from build123d import *

# Parameters (mm, degrees)
SKETCH1_R           = 12.5
SKETCH1_R_2         = 5
BOSS_EXTRUDE1_DEPTH = 15
SKETCH2_R           = 15
SKETCH2_R_2         = 12.5
BOSS_EXTRUDE2_DEPTH = 10
RIB1_REACH          = 70.119
SKETCH3_WALL_W      = 146.04901068
SKETCH3_WALL_H      = 3
CIRPATTERN1_COUNT   = 3


with BuildPart() as part:
    # Sketch1 → Boss-Extrude1 (new body)
    with BuildSketch(Plane(origin=(0, 0, 0), x_dir=(0, 0, -1), z_dir=(1, 0, 0))):
        with BuildLine():
            Line((-41.109265282, -12.912706879), (-8.609265282, 42.087293121))
            ThreePointArc((-8.609265282, 42.087293121), (0, 47), (8.609265282, 42.087293121))
            Line((8.609265282, 42.087293121), (41.109265282, -12.912706879))
            ThreePointArc((41.109265282, -12.912706879), (41.185416835, -22.956161256), (32.5, -28))
            Line((32.5, -28), (-32.5, -28))
            ThreePointArc((-32.5, -28), (-41.185416835, -22.956161256), (-41.109265282, -12.912706879))
        make_face()
        Circle(SKETCH1_R, mode=Mode.SUBTRACT)
        with Locations((0, 37)):
            Circle(SKETCH1_R_2, mode=Mode.SUBTRACT)
        with Locations((32.5, -18)):
            Circle(SKETCH1_R_2, mode=Mode.SUBTRACT)
        with Locations((-32.5, -18)):
            Circle(SKETCH1_R_2, mode=Mode.SUBTRACT)
    extrude(amount=BOSS_EXTRUDE1_DEPTH)

    # Sketch2 → Boss-Extrude2 (add)
    with BuildSketch(Plane(origin=(15, 0, 0), x_dir=(0, 0, -1), z_dir=(1, 0, 0))):
        Circle(SKETCH2_R)
        Circle(SKETCH2_R_2, mode=Mode.SUBTRACT)
    extrude(amount=BOSS_EXTRUDE2_DEPTH)

    # Sketch3 wall → Rib1 (add, up to next)
    with BuildSketch(Plane(origin=(17.5, 18, 0), x_dir=(-0.640184399664, 0.768221279597, 0), z_dir=(-0.768221279597, -0.640184399664, 0)), mode=Mode.PRIVATE) as rib1_sk1:
        Rectangle(SKETCH3_WALL_W, SKETCH3_WALL_H)
    rib1_tool1 = extrude(rib1_sk1.sketch, amount=RIB1_REACH, mode=Mode.PRIVATE) - part.part
    rib1 = rib1_tool1.solids().sort_by_distance((17.5, 18, 0))[0]
    add(rib1)

    # CirPattern1: Rib1 ×3 about axis
    cirpattern1_axis = Axis((0, 0, 0), (1, 0, 0))
    for i in range(1, CIRPATTERN1_COUNT):
        add(rib1.rotate(cirpattern1_axis, i * 360 / CIRPATTERN1_COUNT))


solid = part.part
Verification items for the finished model (mm, model axes). A direction names the side the tool comes from. Give positions to 0.01 mm unless a question says otherwise; leave off trailing zeros. Order: outer loops, then holes, each group sorted by start corner. A loop starts at its lowest first (then second) coordinate and runs counter-clockwise, first axis right, second up. Notation, with made-up numbers: M 31.25,-18 L 49.25,-18 A26 ccw 49.25,8 Z; hole C -27,-12.75 d10. An arc over 180 degrees is marked long. Use one line per item in the form item = value. Start each with the question number.
Q1. Section check C-C (x = 12.25). Enter the section's corners in (y, z).
Q2. Section check B-B (z = 35.5). Enter the section's corners in (x, y), then the cut area to 3 significant figures.
Q3. Mould release check, pull along Y, two halves, no side actions. Record for faces 1 (the flat face through (7.395, 14.972, -24.632)), 2 (the flat face through (7, -28, 0)), 3 (the flat face through (16.758, -7.324, 15.685)): +Y half, -Y half, draft (parallel to the pull), parting line (faces both ways), or undercut.
Q4. Go/stop test with flat-tipped pins: pin 1 Ø13 at (y, z) = (37, 0) entering from +X; pin 2 Ø15 at (y, z) = (0, 0) entering from -X; pin 3 Ø5 at (x, y) = (14, -14.5) entering from +Z; pin 4 Ø4 at (x, y) = (16.5, 17.5) entering from -Z. Record where each tip stops, or that it passes through.
Q5. Access from +Z, -Z, +X, -X, +Y, -Y to the whole of each face (thin tool, end or side, straight path). Record for faces 4 (the flat face through (17, 17, 1.5)), 5 (the flat face through (16.758, -7.324, -15.685)), 6 (the flat face through (15, -15, 9)), 7 (the flat face through (17.567, -8.942, 15.53)), 8 (the flat face through (16.758, -9.922, 14.185)).
Q6. Section check D-D (y = 36). Enter the section's corners in (x, z), then the cut area to 3 significant figures.
Q7. Scan lines: line 1 along Z through (x, y) = (16.5, -7); line 2 along X through (y, z) = (24, 7.5); line 3 along Y through (x, z) = (6.25, 32.5). Record each from-to range of solid material in increasing order. Write a range as [from, to].
Q8. Section check A-A (y = -18). Enter the section's corners in (x, z).
Evaluation:
q1.outline = M -28,-32.5 A10 ccw -12.91,-41.11 L 42.09,-8.61 A10 ccw 42.09,8.61 L -12.91,41.11 A10 ccw -28,32.5 Z; hole C -18,-32.5 d10; hole C -18,32.5 d10; hole C 0,0 d25; hole C 37,0 d10
q2.outline = M 0,-27.54 L 15,-27.54 L 15,-22 L 0,-22 Z; M 0,-14 L 15,-14 L 15,-3.42 L 0,-3.42 Z
q2.area = 242 mm2
q3.face_1 = +Y half
q3.face_2 = -Y half
q3.face_3 = undercut
q4.pin_1 = 15
q4.pin_2 = through
q4.pin_3 = 42.45
q4.pin_4 = -23.92
q5.face_4 = +Z, +X, +Y
q5.face_5 = -Z, +X
q5.face_6 = +X
q5.face_7 = +Z, +X, -Y
q5.face_8 = +X, -Y
q6.outline = M 0,-12.21 L 15,-12.21 L 15,-4.9 L 0,-4.9 Z; M 0,4.9 L 15,4.9 L 15,12.21 L 0,12.21 Z
q6.area = 219 mm2
q7.line_1 = [-15.12, -10.36], [10.36, 15.12]
q7.line_2 = [0, 15]
q7.line_3 = [-28, -23], [-13, 1.66]
q8.outline = M 0,-42.5 L 15,-42.5 L 15,-37.5 L 0,-37.5 Z; M 0,-27.5 L 15,-27.5 L 15,27.5 L 0,27.5 Z; M 0,37.5 L 15,37.5 L 15,42.5 L 0,42.5 Z
